Here's how the part is built. I have some questions about the finished solid (model axes, mm). Face numbers are marked on the shaded views. A direction names the side the tool comes from. Round coordinates to 2 decimals unless told otherwise and drop trailing zeros. Loops run counter-clockwise (first coordinate to the right, second up) from the corner with the lowest first, then second, coordinate; pieces in that order, holes last. Notation, with made-up numbers: M 45.5,47 L 93.5,47 A34 cw 93.5,83 Z; hole C -9,38 d1. An arc over 180 degrees is marked long. Write each question's results on one line, items separated by ' | '. Start each with the question number.
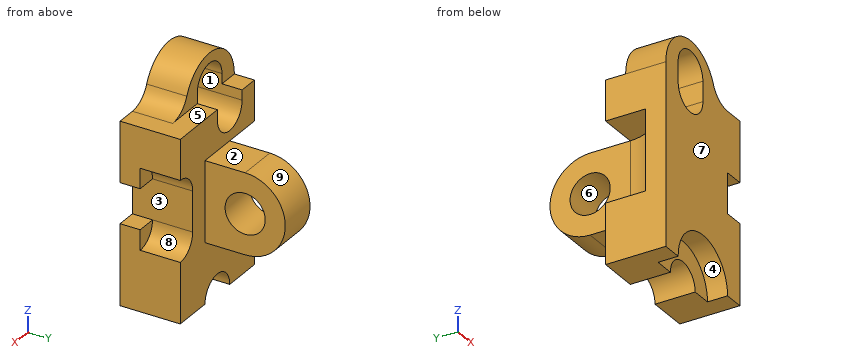
```python
from build123d import *

# Parameters (mm, degrees)
SKETCH1_W           = 6
SKETCH1_H           = 3
BOSS_EXTRUDE1_DEPTH = 9
BOSS_EXTRUDE2_DEPTH = 2
CUT_EXTRUDE1_DEPTH  = 2.5
SKETCH4_W           = 1
SKETCH4_H           = 2
CUT_EXTRUDE2_DEPTH  = 1
CUT_EXTRUDE3_DEPTH  = 2
CUT_EXTRUDE4_DEPTH  = 1
CUT_EXTRUDE5_DEPTH  = 4
SKETCH8_W           = 2
SKETCH8_H           = 4
BOSS_EXTRUDE3_DEPTH = 2
BOSS_EXTRUDE4_DEPTH = 2
SKETCH10_R          = 1
CUT_EXTRUDE6_DEPTH  = 5
SKETCH11_W          = 2
SKETCH11_H          = 4
CUT_EXTRUDE7_DEPTH  = 2
BOSS_EXTRUDE5_DEPTH = 4


with BuildPart() as part:
    # Sketch1 → Boss-Extrude1 (new body)
    with BuildSketch(Plane.XY):
        Rectangle(SKETCH1_W, SKETCH1_H)
    extrude(amount=BOSS_EXTRUDE1_DEPTH)

    # Sketch2 → Boss-Extrude2 (add)
    with BuildSketch(Plane.XZ.offset(1.5)):
        with BuildLine():
            Line((2, 9), (-3, 9))
            ThreePointArc((-3, 9), (-1.39223227, 10.961161351), (0.846153846, 9.769230769))
            ThreePointArc((0.846153846, 9.769230769), (1.306624755, 9.209937132), (2, 9))
        make_face()
    extrude(amount=-BOSS_EXTRUDE2_DEPTH)

    # Sketch3 → Cut-Extrude1 (cut, symmetric)
    with BuildSketch(Plane(origin=(0, 0.5, 0), x_dir=(1, 0, 0), z_dir=(0, 1, 0))):
        with BuildLine():
            Line((-2, -9.5), (-2, -8.5))
            ThreePointArc((-2, -8.5), (-1, -7.5), (0, -8.5))
            Line((0, -8.5), (0, -9.5))
            ThreePointArc((0, -9.5), (-1, -10.5), (-2, -9.5))
        make_face()
    extrude(amount=CUT_EXTRUDE1_DEPTH, both=True, mode=Mode.SUBTRACT)

    # Sketch4 → Cut-Extrude2 (cut)
    with BuildSketch(Plane.XZ.offset(1.5)):
        with Locations((2.5, 5)):
            Rectangle(SKETCH4_W, SKETCH4_H)
    extrude(amount=-CUT_EXTRUDE2_DEPTH, mode=Mode.SUBTRACT)

    # Sketch5 → Cut-Extrude3 (cut)
    with BuildSketch(Plane(origin=(0, 1.5, 0), x_dir=(1, 0, 0), z_dir=(0, 1, 0))):
        with BuildLine():
            Line((4, -4), (4, -6))
            ThreePointArc((4, -6), (3, -7), (2, -6))
            Line((2, -6), (2, -4))
            ThreePointArc((2, -4), (3, -3), (4, -4))
        make_face()
    extrude(amount=-CUT_EXTRUDE3_DEPTH, mode=Mode.SUBTRACT)

    # Sketch6 → Cut-Extrude4 (cut)
    with BuildSketch(Plane.XZ.offset(1.5)):
        with BuildLine():
            Line((2, 0), (-2, 0))
            ThreePointArc((-2, 0), (0, 2), (2, 0))
        make_face()
    extrude(amount=-CUT_EXTRUDE4_DEPTH, mode=Mode.SUBTRACT)

    # Sketch7 → Cut-Extrude5 (cut, through all)
    with BuildSketch(Plane(origin=(0, 1.5, 0), x_dir=(1, 0, 0), z_dir=(0, 1, 0))):
        with BuildLine():
            Line((-1, 0), (1, 0))
            ThreePointArc((1, 0), (0, -1), (-1, 0))
        make_face()
    extrude(amount=-CUT_EXTRUDE5_DEPTH, mode=Mode.SUBTRACT)

    # Sketch8 → Boss-Extrude3 (add)
    with BuildSketch(Plane(origin=(0, 1.5, 0), x_dir=(1, 0, 0), z_dir=(0, 1, 0))):
        with Locations((0, -5)):
            Rectangle(SKETCH8_W, SKETCH8_H)
    extrude(amount=BOSS_EXTRUDE3_DEPTH)

    # Sketch9 → Boss-Extrude4 (add)
    with BuildSketch(Plane(origin=(1, 0, 0), x_dir=(0, 0, -1), z_dir=(1, 0, 0))):
        with BuildLine():
            Line((-3, 3.5), (-7, 3.5))
            ThreePointArc((-7, 3.5), (-5, 5.5), (-3, 3.5))
        make_face()
    extrude(amount=-BOSS_EXTRUDE4_DEPTH)

    # Sketch10 → Cut-Extrude6 (cut, through all)
    with BuildSketch(Plane(origin=(1, 0, 0), x_dir=(0, 0, -1), z_dir=(1, 0, 0))):
        with Locations((-5, 3.5)):
            Circle(SKETCH10_R)
    extrude(amount=-CUT_EXTRUDE6_DEPTH, mode=Mode.SUBTRACT)

    # Sketch11 → Cut-Extrude7 (cut)
    with BuildSketch(Plane(origin=(0, 1.5, 0), x_dir=(1, 0, 0), z_dir=(0, 1, 0))):
        with Locations((-2, -5)):
            Rectangle(SKETCH11_W, SKETCH11_H)
    extrude(amount=-CUT_EXTRUDE7_DEPTH, mode=Mode.SUBTRACT)

    # Sketch12 → Boss-Extrude5 (add)
    with BuildSketch(Plane.XY.offset(3)):
        with BuildLine():
            ThreePointArc((-1, 1.5), (-1.585786438, 0.085786438), (-3, -0.5))
            Line((-3, -0.5), (-1, -0.5))
            Line((-1, -0.5), (-1, 1.5))
        make_face()
    extrude(amount=BOSS_EXTRUDE5_DEPTH)


solid = part.part
```
1. I want a section at B-B on y = 3.25. List the corners of the cut face in (x, z) for me, plus the area to 3 significant figures.
2. I want a section at A-A on z = 5. List the corners of the cut face in (x, y) for me, plus the area to 3 significant figures.
3. If we mould it in two halves opening along Y, with no side actions, what happens to the marked faces 6, 7, 8 and 9? For each: released by +Y, released by -Y, zero draft, split by the parting line, or undercut.
4. I need wall thicknesses on line 1 along Y through (x, z) = (0.25, 5); line 2 along X through (y, z) = (4.5, 3.75); line 3 along Y through (x, z) = (1, 1.5). Which ranges of each line are inside material? Lowest first, please.
5. I want a section at D-D on z = 0.75. List the corners of the cut face in (x, y) for me.
6. For pin 1 (1.2 mm diameter, centred on y = 3, z = 4.5, fed in from +X); pin 2 (0.8 mm diameter, centred on x = 2.5, z = 6.5, fed in from +Y); pin 3 (0.5 mm diameter, centred on x = 2.5, y = -1, fed in from +Z), each with a flat end and sliding along its axis, tell me the tip position at first contact or that it passes through.
7. I want a section at C-C on y = -1. List the corners of the cut face in (x, z) for me, plus the area to 3 significant figures.
8. Which directions (+Z, -Z, +X, -X, +Y, -Y) give clear straight access to the entire face, cutting with the end or side of a thin tool? Please do the marked faces 1, 2, 3, 4 and 5.
Outcome:
1) outline: M -1,3 L 1,3 L 1,4.03 L -1,4.03 Z; M -1,5.97 L 1,5.97 L 1,7 L -1,7 Z | area: 4.13 mm2
2) outline: M -3,-1.5 L 2,-1.5 L 2,1.5 L 1,1.5 L 1,2.5 L -1,2.5 L -1,1.5 A2 cw -3,-0.5 Z; M -1,4.5 L 1,4.5 L 1,5.5 L -1,5.5 Z | area: 15.9 mm2
3) face 6: undercut | face 7: released by -Y | face 8: zero draft | face 9: released by +Y
4) line 1: -1.5 to 2.5, 4.5 to 5.5 | line 2: -1 to 1 | line 3: -0.5 to 1.5
5) outline: M -3,-1.5 L -1.85,-1.5 L -1.85,-0.5 L -0.66,-0.5 L -0.66,1.5 L -3,1.5 Z; M 0.66,-0.5 L 1.85,-0.5 L 1.85,-1.5 L 3,-1.5 L 3,1.5 L 0.66,1.5 Z
6) pin 1: x = 1 | pin 2: y = 1.5 | pin 3: z = 9
7) outline: M -3,0 L -2,0 A2 cw 2,0 L 3,0 L 3,4 L 2,4 L 2,6 L 3,6 L 3,9 L 2,9 A1.25 cw 0.85,9.77 A2 ccw -3,9 Z; hole M -2,8.5 A1 ccw 0,8.5 L 0,9.5 A1 ccw -2,9.5 Z | area: 47.0 mm2
8) face 1: +Y, -Y | face 2: +Z, +X, -X, +Y | face 3: +X, +Y, -Y | face 4: -Z, -Y | face 5: +Z, +X, +Y
